The figure shows three views and two pictorial views of one solid part (mm, origin at its lowest corner). Answer the questions. A direction names the side the tool comes from. Coordinates: 2 decimals unless noted, no trailing zeros. Order: outer loops, then holes, each group sorted by start corner. A loop starts at its lowest first (then second) coordinate and runs counter-clockwise, first axis right, second up.
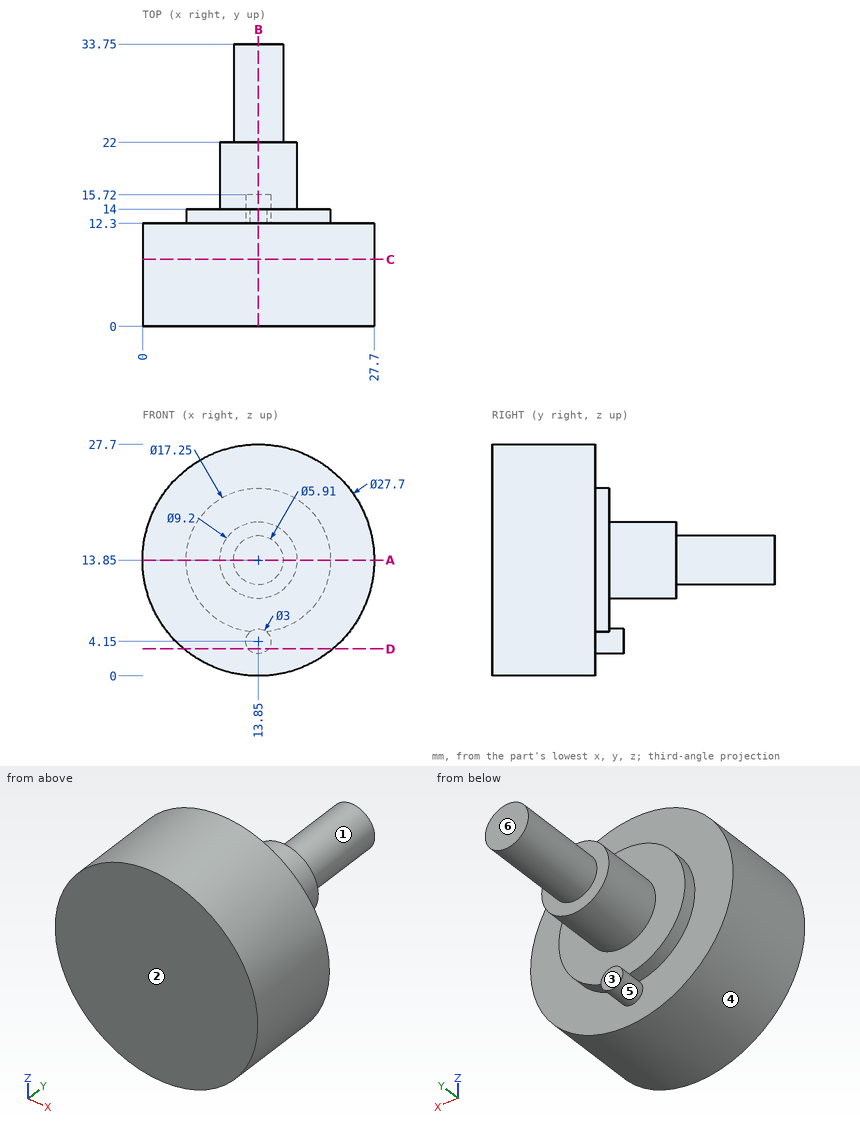
Q1. The part is cut by section C-C, the plane y = 8. Determine the outline of the cut face in (x, z), then the cut area to 3 significant figures.
Q2. Determine the mould class of the marked faces 4, 5 and 6 for opening direction Z: +Z half, -Z half, draft (parallel to the pull), parting line (faces both ways), or undercut.
Q3. Which of the six approach directions +Z, -Z, +X, -X, +Y, -Y give full straight-line access (tool end or side, diameter ignored) to the marked faces 1, 2 and 3?
Q4. Each of these flat-tipped pins is pushed along its axis until it touches: P1, Ø2, axis at x = 13, y = 9.5, coming from the -Z side; P2, Ø5, axis at x = 21, y = 28.5, coming from the -Z side; P3, Ø6, axis at x = 24.5, z = 3, coming from the +Y side; P4, Ø6, axis at x = 8.5, y = 14.5, coming from the -Z side. Where does it stop, or does it pass through?
Q5. The part is cut by section A-A, the plane z = 13.85. Determine the outline of the cut face in (x, y) (3 decimals), then the cut area to 3 significant figures.
Q6. Straight lines are drawn through the part: L1, parallel to Y at x = 3.75, z = 14.5; L2, parallel to Y at x = 18, z = 7.75; L3, parallel to Z at x = 16, y = 11. For each, find the intervals that lie inside material, in ascending order.
Q7. The part is cut by section D-D, the plane z = 3.25. Determine the outline of the cut face in (x, y).
Q8. The part is cut by section B-B, the plane x = 13.85. Determine the outline of the cut face in (y, z) (3 decimals).
Computed values:
1. outline: circle Ø27.7 at (13.85, 13.85)
1. area: 603 mm2
2. face 4: parting line
2. face 5: undercut
2. face 6: draft
3. face 1: +Y
3. face 2: +Z, -Z, +X, -X, -Y
3. face 3: -Z, +X, -X, +Y
4. P1: stops at z = 0
4. P2: passes through
4. P3: stops at y = 12.3
4. P4: stops at z = 0.4
5. outline: (0, 0) - (27.7, 0) - (27.7, 12.3) - (22.475, 12.3) - (22.475, 14) - (18.45, 14) - (18.45, 22) - (16.805, 22) - (16.805, 33.75) - (10.895, 33.75) - (10.895, 22) - (9.25, 22) - (9.25, 14) - (5.225, 14) - (5.225, 12.3) - (0, 12.3) - close
5. area: 513 mm2
6. L1: y = 0 to 12.3
6. L2: y = 0 to 14
6. L3: z = 0.17 to 27.53
7. outline: (4.94, 0) - (22.76, 0) - (22.76, 12.3) - (15.05, 12.3) - (15.05, 15.72) - (12.65, 15.72) - (12.65, 12.3) - (4.94, 12.3) - close
8. outline: (0, 0) - (12.3, 0) - (12.3, 2.65) - (15.72, 2.65) - (15.72, 5.65) - (14, 5.65) - (14, 9.25) - (22, 9.25) - (22, 10.895) - (33.75, 10.895) - (33.75, 16.805) - (22, 16.805) - (22, 18.45) - (14, 18.45) - (14, 22.475) - (12.3, 22.475) - (12.3, 27.7) - (0, 27.7) - close
